```python
from build123d import *

# Parameters (mm, degrees)
EXTRUDE1_DEPTH                 = 5
LPATTERN1_COUNT                = 2
LPATTERN1_PITCH                = 50
LPATTERN1_COUNT_DIR2           = 2
LPATTERN1_PITCH_DIR2           = 25
SKETCH5_W                      = 10
SKETCH5_H                      = 5
EXTRUDE2_DEPTH                 = 50
SKETCH6_W                      = 10
SKETCH6_H                      = 7
EXTRUDE3_DEPTH                 = 10
F_1_8_0_125_DIAMETER_HOLE1_D   = 3.175
F_1_16_0_0625_DIAMETER_HOLE1_D = 1.5875
F_8_32_TAPPED_HOLE1_D          = 3.4544


with BuildPart() as part:
    # Sketch1 → Extrude1 (new body)
    with BuildSketch(Plane(origin=(0, 0, 0), x_dir=(1, 0, 0), z_dir=(0, 1, 0))):
        Polygon((-20, -7.5), (-20, 18.5), (-31, 18.5), (-31, -18.5), (31, -18.5), (31, 18.5), (20, 18.5), (20, -7.5), align=None)
    extrude(amount=EXTRUDE1_DEPTH)

    # Sketch4 → M6 Clearance Hole1 (revolve, cut)
    with BuildSketch(Plane(origin=(-25, 5, -12.5), x_dir=(0, 0, 1), z_dir=(1, 0, 0))):
        Polygon((0, 0), (0, 11.982840043), (3.3, 10), (3.3, 0), align=None)
    m6_clearance_hole1 = revolve(axis=Axis((-25, 11.35, -12.5), (0, -1, 0)), mode=Mode.SUBTRACT)

    # LPattern1: M6 Clearance Hole1 2 × 2
    with Locations(*[(i * LPATTERN1_PITCH, 0, j * LPATTERN1_PITCH_DIR2) for i in range(LPATTERN1_COUNT) for j in range(LPATTERN1_COUNT_DIR2) if (i, j) != (0, 0)]):
        add(m6_clearance_hole1, mode=Mode.SUBTRACT)

    # Sketch5 → Extrude2 (add)
    with BuildSketch(Plane.XY.offset(18.5)):
        with Locations((0, 2.5)):
            Rectangle(SKETCH5_W, SKETCH5_H)
    extrude(amount=EXTRUDE2_DEPTH)

    # Sketch6 → Extrude3 (add)
    with BuildSketch(Plane(origin=(0, 5, 0), x_dir=(1, 0, 0), z_dir=(0, 1, 0))):
        with Locations((0, -65)):
            Rectangle(SKETCH6_W, SKETCH6_H)
    extrude(amount=EXTRUDE3_DEPTH)

    # 1/8 (0.125) Diameter Hole1 (through all)
    with Locations(Plane(origin=(0, 12, 61.5), x_dir=(-1, 0, 0), z_dir=(0, 0, -1))):
        with Locations((0, 0)):
            Hole(F_1_8_0_125_DIAMETER_HOLE1_D / 2)

    # 1/16 (0.0625) Diameter Hole1 (through all)
    with Locations(Plane(origin=(0, 13.25, 61.5), x_dir=(-1, 0, 0), z_dir=(0, 0, -1))):
        with Locations((0, 0)):
            Hole(F_1_16_0_0625_DIAMETER_HOLE1_D / 2)

    # #8-32 Tapped Hole1 (through all)
    with Locations(Plane(origin=(0, 0, 65), x_dir=(0, 0, -1), z_dir=(0, -1, 0))):
        with Locations((0, 0)):
            Hole(F_8_32_TAPPED_HOLE1_D / 2)


solid = part.part
```
Verification items for the finished model (mm, model axes). A direction names the side the tool comes from. Give positions to 0.01 mm unless a question says otherwise; leave off trailing zeros. Order: outer loops, then holes, each group sorted by start corner. A loop starts at its lowest first (then second) coordinate and runs counter-clockwise, first axis right, second up. Notation, with made-up numbers: M -14.5,69 L -1.5,69 A17 cw -1.5,101 Z; hole C 56.25,38 d4. An arc over 180 degrees is marked long. Return JSON: item names as keys, results as strings. Group by question number.
1) Section check A-A on x = -25. Record the cut outline in (y, z), and give its area (3 significant figures).
2) Section check B-B on z = 12.5. Record the cut outline in (x, y), and give its area (3 significant figures).
3) Section check D-D on z = -12.5. Record the cut outline in (x, y).
4) Mould release check, pull along Y, two halves, no side actions. Record for faces 5 (the face through (18, 2, 18.5)), 6 (the face through (-0.058, 10.414, 67.423)), 7 (the face through (0, 5, 15)): pulls with the +Y half, pulls with the -Y half, needs draft (parallel to the pull), parting line crosses it, or undercut.
5) Go/stop test with flat-tipped pins: pin 1 Ø8.5 at (x, z) = (-25, -12.5) entering from +Y; pin 2 Ø1.5 at (y, z) = (2.5, 33.5) entering from +X; pin 3 Ø5.5 at (x, y) = (-14, 3) entering from +Z. Record where each tip stops, or that it passes through.
6) Section check C-C on y = 12. Record the cut outline in (x, z).
7) Access from +Z, -Z, +X, -X, +Y, -Y to the whole of each face (thin tool, end or side, straight path). Record for faces 1 (the face through (5, 4, 49)), 2 (the face through (-5, 4, 49)), 3 (the face through (-20, 2, -5)), 4 (the face through (0, 10, 61.5)).
8) Scan lines: line 1 (X direction, y = 2.55, z = 12.5); line 2 (X direction, y = 1.9, z = -12.5); line 3 (Z direction, x = -25, y = 2). Record each from-to range of solid material in increasing order.
Answer block:
{
 "1": {"outline": "M 0,-18.5 L 5,-18.5 L 5,-15.8 L 0,-15.8 Z; M 0,-9.2 L 5,-9.2 L 5,9.2 L 0,9.2 Z; M 0,15.8 L 5,15.8 L 5,18.5 L 0,18.5 Z", "area": "119 mm^2"},
 "2": {"outline": "M -31,0 L -28.3,0 L -28.3,5 L -31,5 Z; M -21.7,0 L 21.7,0 L 21.7,5 L -21.7,5 Z; M 28.3,0 L 31,0 L 31,5 L 28.3,5 Z", "area": "244 mm^2"},
 "3": {"outline": "M -31,0 L -28.3,0 L -28.3,5 L -31,5 Z; M -21.7,0 L -20,0 L -20,5 L -21.7,5 Z; M 20,0 L 21.7,0 L 21.7,5 L 20,5 Z; M 28.3,0 L 31,0 L 31,5 L 28.3,5 Z"},
 "4": {"face 5": "needs draft", "face 6": "undercut", "face 7": "pulls with the +Y half"},
 "5": {"pin 1": "stops at y = 5", "pin 2": "stops at x = 5", "pin 3": "stops at z = 18.5"},
 "6": {"outline": "M -5,61.5 L -1.59,61.5 L -1.59,64.32 A1.73 cw -1.59,65.68 L -1.59,68.5 L -5,68.5 Z; M 1.59,61.5 L 5,61.5 L 5,68.5 L 1.59,68.5 L 1.59,65.68 A1.73 cw 1.59,64.32 Z"},
 "7": {"face 1": "+Z, +X, +Y, -Y", "face 2": "+Z, -X, +Y, -Y", "face 3": "-Z, +Y, -Y", "face 4": "-Z, +X, -X, +Y"},
 "8": {"line 1": "x = -31 to -28.3, -21.7 to 21.7, 28.3 to 31", "line 2": "x = -31 to -28.3, -21.7 to -20, 20 to 21.7, 28.3 to 31", "line 3": "z = -18.5 to -15.8, -9.2 to 9.2, 15.8 to 18.5"}
}
